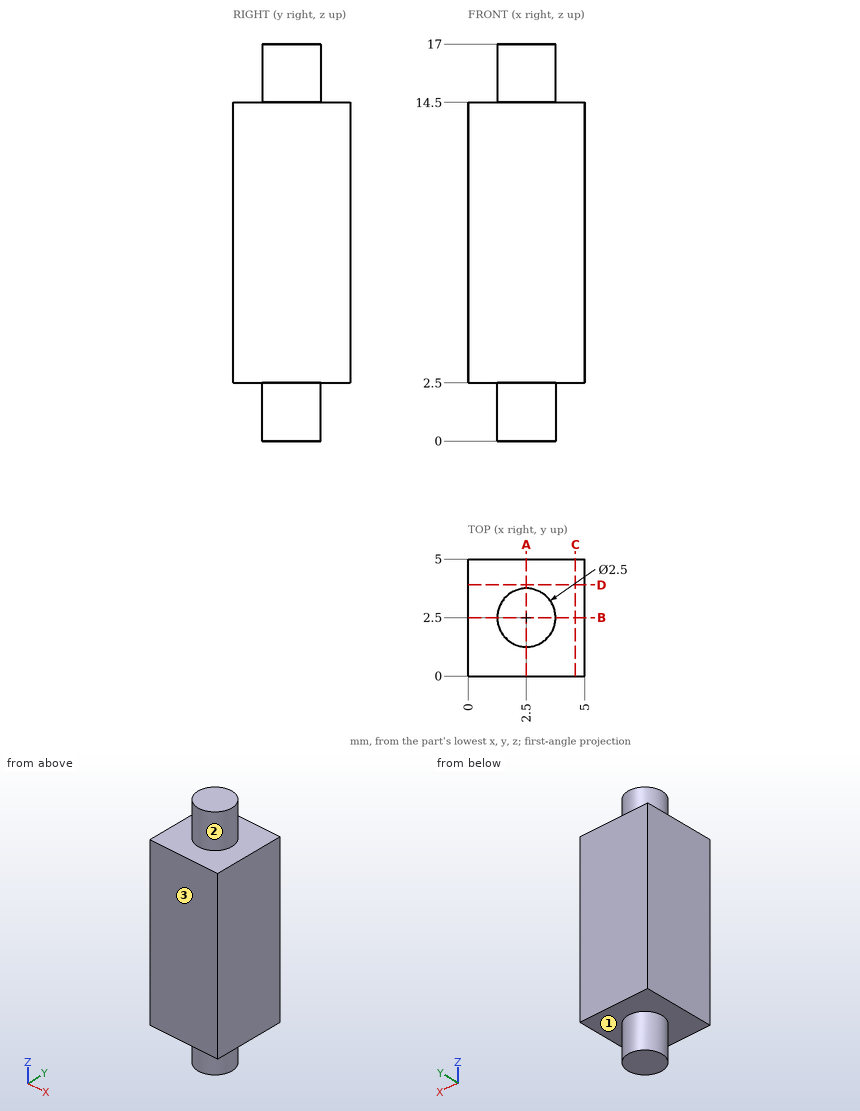
The figure shows three views and two pictorial views of one solid part (mm, origin at its lowest corner). Answer the questions. A direction names the side the tool comes from. Coordinates: 2 decimals unless noted, no trailing zeros. Write each loop counter-clockwise with the first axis right and the second up, starting at its lowest first coordinate (ties: lowest second). Pieces come first, ordered by that corner, then holes. Notation, with made-up numbers: M -1,34.25 L 47,34.25 A27 cw 47,61.25 Z; hole C -15,43 d3. An arc over 180 degrees is marked long. Answer as CSV lines item,"result". Start each with the question number.
Item 1: Section A-A on x = 2.5 is taken. Write down the section's boundary in (y, z).
Item 2: Consider L1, parallel to Z at x = 4.75, y = 2.45; L2, parallel to Y at x = 2.4, z = 16; L3, parallel to Y at x = 1.8, z = 0.5. Determine where each line is inside the solid, lowest interval first.
Item 3: A tool of negligible diameter and unlimited length cuts with its end or side. For the marked faces 1, 2 and 3, from which of +Z, -Z, +X, -X, +Y, -Y can it reach the whole face along a straight path? Write none if from no direction.
Item 4: Section C-C on x = 4.6 is taken. Write down the section's boundary in (y, z).
Checks:
1,outline,"M 0,2.5 L 1.25,2.5 L 1.25,0 L 3.75,0 L 3.75,2.5 L 5,2.5 L 5,14.5 L 3.75,14.5 L 3.75,17 L 1.25,17 L 1.25,14.5 L 0,14.5 Z"
2,L1,"z = 2.5 to 14.5"
2,L2,"y = 1.25 to 3.75"
2,L3,"y = 1.46 to 3.54"
3,face 1,"-Z"
3,face 2,"+Z"
3,face 3,"+Z, -Z, +X, -X, -Y"
4,outline,"M 0,2.5 L 5,2.5 L 5,14.5 L 0,14.5 Z"
